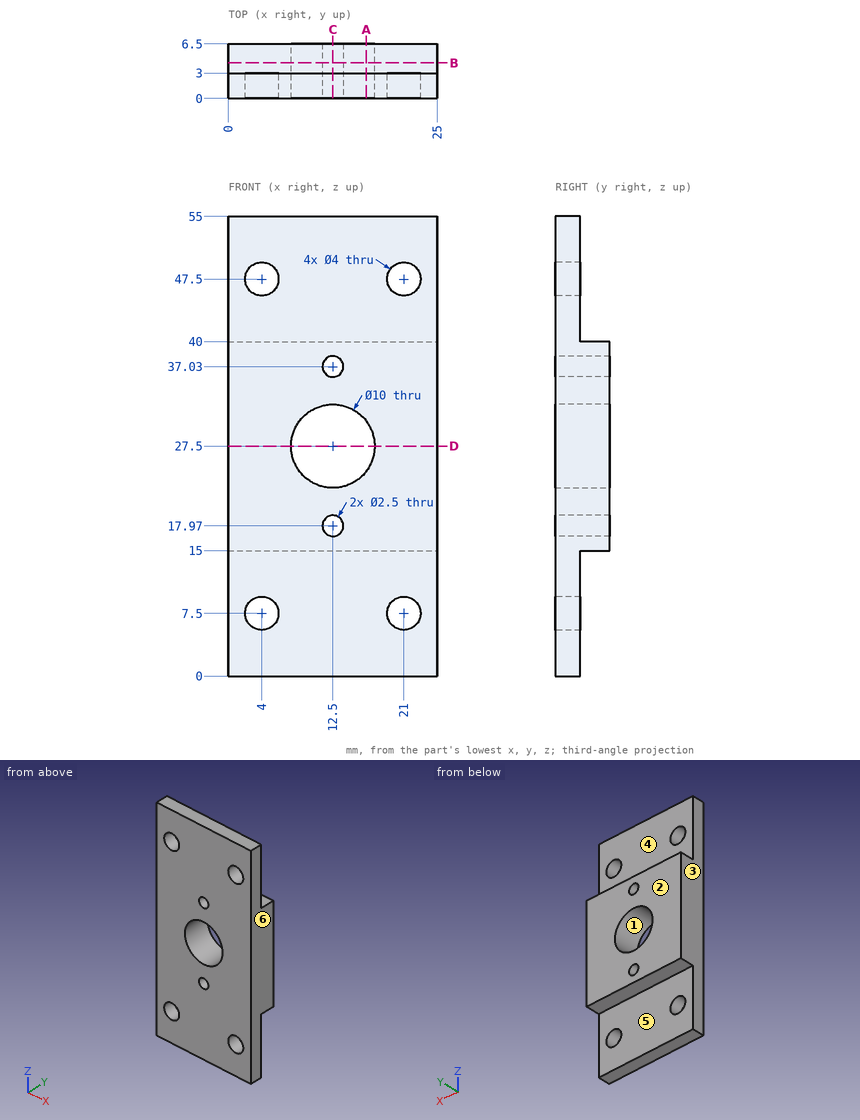
Job drawing, mm, ordinate dimensions from the low corner. One solid piece. A direction names the side the tool comes from. Coordinates: 2 decimals unless noted, no trailing zeros. Order: outer loops, then holes, each group sorted by start corner. A loop starts at its lowest first (then second) coordinate and runs counter-clockwise, first axis right, second up. Notation, with made-up numbers: M 26,46.25 L 39,46.25 A11 cw 39,58.25 Z; hole C 62.5,11.5 d10. An arc over 180 degrees is marked long. One line per question, with ' | ' between items.
Q1. Slice it at B-B (y = 4.25). Give the cut face in (x, z), and give its area (3 significant figures).
A:
outline: M 0,15 L 25,15 L 25,40 L 0,40 Z; hole C 12.5,27.5 d10; hole C 12.5,17.97 d2.5; hole C 12.5,37.03 d2.5 | area: 537 mm^2
Q2. Slice it at A-A (x = 16.5). Give the cut face in (y, z).
A:
outline: M 0,0 L 3,0 L 3,15 L 6.5,15 L 6.5,24.5 L 0,24.5 Z; M 0,30.5 L 6.5,30.5 L 6.5,40 L 3,40 L 3,55 L 0,55 Z
Q3. Pin check, flat tips, straight feed: P1, Ø2, axis at x = 12.5, z = 17.97, coming from the +Y side; P2, Ø1, axis at x = 12.5, y = 5.5, coming from the +Z side; P3, Ø6, axis at x = 10, z = 44.5, coming from the +Y side; P4, Ø3, axis at x = 13, y = 5, coming from the -Z side. Stop position of each tip, or through.
A:
P1: passes through | P2: stops at z = 40 | P3: stops at y = 3 | P4: stops at z = 15
Q4. 3-axis set-ups, long thin cutter, end or side, ignore diameter. For the marked faces 4, 5 and 6: which of +Z, -Z, +X, -X, +Y, -Y reach the whole face in a straight line?
A:
face 4: +Z, +X, -X, +Y | face 5: -Z, +X, -X, +Y | face 6: +Z, -Z, +X, +Y, -Y
Q5. Drill centre lines: line 1 (X direction, y = 1.2, z = 47.5); line 2 (Z direction, x = 20, y = 2.5); line 3 (Y direction, x = 16.75, z = 7). Where is each one in solid material? Low to high.
A:
line 1: x = 0 to 2, 6 to 19, 23 to 25 | line 2: z = 0 to 5.77, 9.23 to 45.77, 49.23 to 55 | line 3: y = 0 to 3
Q6. Slice it at C-C (x = 12.5). Give the cut face in (y, z), and give its area (3 significant figures).
A:
outline: M 0,0 L 3,0 L 3,15 L 6.5,15 L 6.5,16.72 L 0,16.72 Z; M 0,19.22 L 6.5,19.22 L 6.5,22.5 L 0,22.5 Z; M 0,32.5 L 6.5,32.5 L 6.5,35.78 L 0,35.78 Z; M 0,38.28 L 6.5,38.28 L 6.5,40 L 3,40 L 3,55 L 0,55 Z | area: 155 mm^2
Q7. Slice it at D-D (z = 27.5). Give the cut face in (x, y).
A:
outline: M 0,0 L 7.5,0 L 7.5,6.5 L 0,6.5 Z; M 17.5,0 L 25,0 L 25,6.5 L 17.5,6.5 Z
Q8. Two-plate mould, pull along X, no slides. Class the marked faces 1, 2 and 3: +X half, -X half, draft (parallel to the pull), parting line (faces both ways), or undercut.
A:
face 1: undercut | face 2: draft | face 3: -X half
